The model under review builds one solid part; all positions refer to its coordinate system, in mm. Give positions to 0.01 mm unless a question says otherwise; leave off trailing zeros. Loops run counter-clockwise (first coordinate to the right, second up) from the corner with the lowest first, then second, coordinate; pieces in that order, holes last. Notation, with made-up numbers: M -9.75,-19.75 L 24.25,-19.75 A30 cw 24.25,6.25 Z; hole C 31,51.25 d3. An arc over 180 degrees is marked long. One line per item, written item: value. Start each with the question number.
Q1. To check wall thickness, follow line 1 along X through (y, z) = (1.75, -65); line 2 along Z through (x, y) = (55, 1.45); line 3 along Z through (x, y) = (-53.5, 1.9). State the ranges of each line that lie inside material, in increasing order. Write a range as from..to.
Q2. Mouldability with a two-part tool opening along X and no side actions: class faces 1 (the face through (65, 1, -90)), 2 (the face through (-56.29, 1.479, -67.024)), 3 (the face through (-1, 3, -1)) as released by +X, released by -X, zero draft, split by the parting line, or undercut.
Q3. We need section B-B on x = -55. Write out the cut boundary in (y, z), plus the area to 3 significant figures.
Q4. We need section A-A on z = -65. Write out the cut boundary in (x, y), plus the area to 3 significant figures.
Q5. For pin 1 (3 mm diameter, centred on x = 55, z = -65, fed in from -Y), flat-tipped, find the tip position at first contact; note if it passes through.
```python
from build123d import *

# Parameters (mm, degrees)
SKETCH1_W            = 140
SKETCH1_H            = 190
BOSS_EXTRUDE1_DEPTH  = 3
M4_CLEARANCE_HOLE1_D = 4.8
CHAMFER1_SIZE        = 10


with BuildPart() as part:
    # Sketch1 → Boss-Extrude1 (new body)
    with BuildSketch(Plane(origin=(0, 0, 0), x_dir=(1, 0, 0), z_dir=(0, 1, 0))):
        Rectangle(SKETCH1_W, SKETCH1_H)
    extrude(amount=BOSS_EXTRUDE1_DEPTH)

    # M4 Clearance Hole1 (through all)
    with Locations(Plane(origin=(0, 3, 0), x_dir=(1, 0, 0), z_dir=(0, 1, 0))):
        with Locations((-55, -85), (55, -85), (-55, 65), (55, 65)):
            Hole(M4_CLEARANCE_HOLE1_D / 2)

    # Chamfer1
    chamfer1_edges = [part.edges().sort_by_distance(p)[0] for p in [
        (-70, 1.5, -95),
        (70, 1.5, -95),
    ]]
    chamfer(chamfer1_edges, length=CHAMFER1_SIZE)


solid = part.part
```
Solved:
1. line 1: -70..-57.4, -52.6..52.6, 57.4..70
1. line 2: -95..-67.4, -62.6..82.6, 87.4..95
1. line 3: -95..-66.87, -63.13..83.13, 86.87..95
2. face 1: released by +X
2. face 2: undercut
2. face 3: zero draft
3. outline: M 0,-95 L 3,-95 L 3,-67.4 L 0,-67.4 Z; M 0,-62.6 L 3,-62.6 L 3,82.6 L 0,82.6 Z; M 0,87.4 L 3,87.4 L 3,95 L 0,95 Z
3. area: 541 mm2
4. outline: M -70,0 L -57.4,0 L -57.4,3 L -70,3 Z; M -52.6,0 L 52.6,0 L 52.6,3 L -52.6,3 Z; M 57.4,0 L 70,0 L 70,3 L 57.4,3 Z
4. area: 391 mm2
5. pin 1: through
